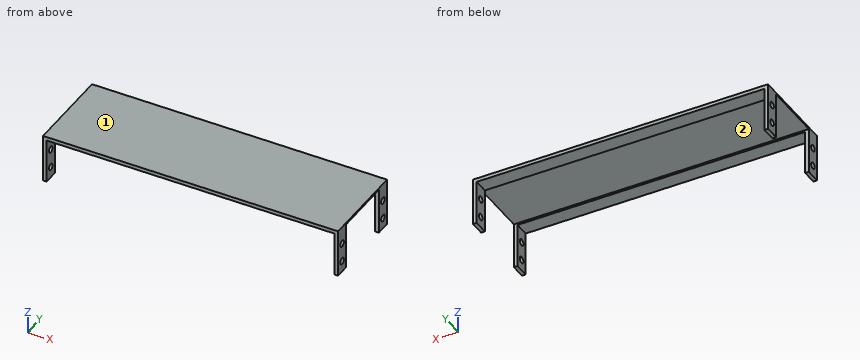
from build123d import *

# Parameters (mm, degrees)
F0_W          = 508
F0_H          = 6.35
F1_DEPTH      = 76.2
F2_W          = 6.35
F2_H          = 76.2
F3_DEPTH      = 76.2
F4_W          = 101.6
F4_H          = 79.375
F5_DEPTH      = 254.001
F5_DEPTH_BACK = 254.001
F6_R          = 5.55625
F7_DEPTH      = 508.001


with BuildPart() as f1:
    # F0 (on Front) → F1 (new body, symmetric)
    with BuildSketch(Plane.XZ):
        Rectangle(F0_W, F0_H)
    extrude(amount=F1_DEPTH, both=True)

    # F2 (on Front) → F3 (join, symmetric)
    with BuildSketch(Plane.XZ):
        with Locations((-250.825, -41.275)):
            Rectangle(F2_W, F2_H)
        with Locations((250.825, -41.275)):
            Rectangle(F2_W, F2_H)
    extrude(amount=F3_DEPTH, both=True)

    # F4 (on Right) → F5 (cut, two sides)
    with BuildSketch(Plane.YZ) as f5_sk:
        with Locations((0, -39.6875)):
            Rectangle(F4_W, F4_H)
    extrude(amount=-F5_DEPTH, mode=Mode.SUBTRACT)
    extrude(f5_sk.sketch, amount=F5_DEPTH_BACK, mode=Mode.SUBTRACT)

    # F6 (on face) → F7 (cut, through all)
    with BuildSketch(Plane.YZ.offset(254)):
        with Locations((-63.5, -27.813)):
            Circle(F6_R)
        with Locations((-63.5, -60.325)):
            Circle(F6_R)
        with Locations((63.5, -27.813)):
            Circle(F6_R)
        with Locations((63.5, -60.325)):
            Circle(F6_R)
    extrude(amount=-F7_DEPTH, mode=Mode.SUBTRACT)


solid = f1.part
The model under review builds one solid part; all positions refer to its coordinate system, in mm. Face numbers are marked on the shaded views. Coordinates: 2 decimals unless noted, no trailing zeros. Loops run counter-clockwise (first coordinate to the right, second up) from the corner with the lowest first, then second, coordinate; pieces in that order, holes last.
(1) Consider section A-A, the plane z = -15.5. Give the boundary of the cut face in (x, y).
Determined:
outline: (-254, -76.2) - (-247.65, -76.2) - (-247.65, -50.8) - (-254, -50.8) - close; (-254, 50.8) - (-247.65, 50.8) - (-247.65, 76.2) - (-254, 76.2) - close; (247.65, -76.2) - (254, -76.2) - (254, -50.8) - (247.65, -50.8) - close; (247.65, 50.8) - (254, 50.8) - (254, 76.2) - (247.65, 76.2) - close
(2) Draft analysis for pull direction Y (two halves, no side actions). For the marked faces 1 and 2, state which applies: +Y half, -Y half, draft (parallel to the pull), parting line (faces both ways), or undercut.
Determined:
face 1: draft
face 2: undercut
(3) Consider section C-C, the plane x = 194. Give the boundary of the cut face in (y, z) (3 decimals).
Determined:
outline: (-76.2, -3.175) - (-50.8, -3.175) - (-50.8, 0) - (50.8, 0) - (50.8, -3.175) - (76.2, -3.175) - (76.2, 3.175) - (-76.2, 3.175) - close
(4) Wall thickness on L1, parallel to Z at x = -252, y = -63 (3 decimals); L2, parallel to Z at x = -252.25, y = -63.5 (3 decimals); L3, parallel to X at y = -57, z = -69: over which ranges is each line inside the solid? List them lowest first.
Determined:
L1: z = -79.375 to -65.859, -54.791 to -33.347, -22.279 to 3.175
L2: z = -79.375 to -65.881, -54.769 to -33.369, -22.257 to 3.175
L3: x = -254 to -247.65, 247.65 to 254
(5) Insertion check: P1, Ø7.5, axis at y = 66.5, z = -26, coming from the -X side; P2, Ø7.5, axis at x = -112.5, y = 58, coming from the -Z side (3 decimals); P3, Ø6, axis at x = 44.5, y = 31, coming from the -Z side. Each pin has a flat end and moves straight along its axis. Give the tip position at first contact, or say it passes through.
Determined:
P1: stops at x = -254
P2: stops at z = -3.175
P3: stops at z = 0
(6) Consider section B-B, the plane y = 63.5. Give the boundary of the cut face in (x, z) (3 decimals), plus the area to 3 significant figures.
Determined:
outline: (-254, -79.375) - (-247.65, -79.375) - (-247.65, -65.881) - (-254, -65.881) - close; (-254, -54.769) - (-247.65, -54.769) - (-247.65, -33.369) - (-254, -33.369) - close; (-254, -22.257) - (-247.65, -22.257) - (-247.65, -3.175) - (247.65, -3.175) - (247.65, -22.257) - (254, -22.257) - (254, 3.175) - (-254, 3.175) - close; (247.65, -79.375) - (254, -79.375) - (254, -65.881) - (247.65, -65.881) - close; (247.65, -54.769) - (254, -54.769) - (254, -33.369) - (247.65, -33.369) - close
area: 3,910 mm2
(7) Consider section D-D, the plane y = 40.5. Give the boundary of the cut face in (x, z) (3 decimals).
Determined:
outline: (-254, 0) - (254, 0) - (254, 3.175) - (-254, 3.175) - close
